from build123d import *

# Parameters (mm, degrees)
EXTRUDE1_DEPTH          = 45
EXTRUDE1_DEPTH_BACK     = 45
SKETCH1_R               = 6
EXTRUDE2_DEPTH          = 41
EXTRUDE2_DEPTH_BACK     = 41
SKETCH2_R               = 6.35
CUT_EXTRUDE1_DEPTH      = 46.887307613
CUT_EXTRUDE1_DEPTH_BACK = 46.887307613
SKETCH3_R               = 4.365


with BuildPart() as part:
    # Sketch1 → Extrude1 (new, two sides: drawn at the far end of the back side and taken through both)
    with BuildSketch(Plane.XY.offset(-EXTRUDE1_DEPTH_BACK)):
        with Locations(Location((0, 0, 0), (0, 0, 180))):
            Circle(SKETCH1_R)
    extrude(amount=EXTRUDE1_DEPTH + EXTRUDE1_DEPTH_BACK)

    # Sketch2 → Extrude2 (add, two sides: drawn at the far end of the back side and taken through both)
    with BuildSketch(Plane.XY.offset(-EXTRUDE2_DEPTH_BACK)):
        with Locations(Location((0, 0, 0), (0, 0, 180))):
            Circle(SKETCH2_R)
    extrude(amount=EXTRUDE2_DEPTH + EXTRUDE2_DEPTH_BACK)

    # Sketch3 → Cut-Extrude1 (cut, two sides: drawn at the far end of the back side and taken through both)
    with BuildSketch(Plane.XY.offset(-CUT_EXTRUDE1_DEPTH_BACK)):
        Circle(SKETCH3_R)
    extrude(amount=CUT_EXTRUDE1_DEPTH + CUT_EXTRUDE1_DEPTH_BACK, mode=Mode.SUBTRACT)


solid = part.part
Work out the finished part from the listing and answer in its coordinate system (mm). A direction names the side the tool comes from. Give positions to 0.01 mm unless a question says otherwise; leave off trailing zeros. Order: outer loops, then holes, each group sorted by start corner. A loop starts at its lowest first (then second) coordinate and runs counter-clockwise, first axis right, second up. Notation, with made-up numbers: (79.25, -10) -> (96.25, -10) arc R22 ccw to (96.25, 12) -> close; hole circle Ø4 at (19.5, 76). An arc over 180 degrees is marked (long way). Answer as a JSON object with one key per item and string values. Group by question number.
1. Section C-C on z = 18.5 is taken. Determine the outline of the cut face in (x, y) (3 decimals), plus the area to 3 significant figures.
2. Section A-A on x = 0 is taken. Determine the outline of the cut face in (y, z) (3 decimals).
3. Consider line 1 along Y through (x, z) = (0, 21.5) (3 decimals); line 2 along Y through (x, z) = (3, -29); line 3 along X through (y, z) = (-4, -31). Determine where each line is inside the solid, lowest interval first. Write a range as [from, to].
4. A tool of negligible diameter and unlimited length cuts with its end or side. For faces 1 (the cylindrical face through (-5.723, -1.802, -43.028)), 2 (the cylindrical face through (-2.93, 5.634, -0.574)), from which of +Z, -Z, +X, -X, +Y, -Y can it reach the whole face along a straight path? Write none if from no direction.
5. Flat-ended cylindrical pins translate along their axes: pin 1 Ø6 at (x, z) = (5, 23) entering from -Y; pin 2 Ø3 at (y, z) = (-2, -12) entering from -X; pin 3 Ø1.5 at (y, z) = (4, 33.5) entering from -X. Find the tip coordinate at first contact, or state that the pin passes through.
6. The mould has two halves that part along X. Classify faces 3 (the cylindrical face through (-5.723, -1.802, 42.972)), 4 (the cylindrical face through (-3.217, 2.95, -0.63)), 5 (the flat face through (3, 4, 45)): released by +X, released by -X, zero draft, split by the parting line, or undercut.
Result sheet:
{
 "1": {"outline": "circle Ø12.7 at (0, 0); hole circle Ø8.73 at (0, 0)", "area": "66.8 mm^2"},
 "2": {"outline": "(-6.35, -41) -> (-6, -41) -> (-6, -45) -> (-4.365, -45) -> (-4.365, 45) -> (-6, 45) -> (-6, 41) -> (-6.35, 41) -> close; (4.365, -45) -> (6, -45) -> (6, -41) -> (6.35, -41) -> (6.35, 41) -> (6, 41) -> (6, 45) -> (4.365, 45) -> close"},
 "3": {"line 1": "y = [-6.35, -4.365], [4.365, 6.35]", "line 2": "y = [-5.6, -3.17], [3.17, 5.6]", "line 3": "x = [-4.93, -1.75], [1.75, 4.93]"},
 "4": {"face 1": "-Z", "face 2": "+Z, -Z"},
 "5": {"pin 1": "stops at y = -6.03", "pin 2": "stops at x = -6.33", "pin 3": "stops at x = -5.46"},
 "6": {"face 3": "split by the parting line", "face 4": "undercut", "face 5": "zero draft"}
}
